Study the drawing (mm; zero at the part's minimum x, y, z) and answer. A direction names the side the tool comes from. Round coordinates to 2 decimals unless told otherwise and drop trailing zeros. Order: outer loops, then holes, each group sorted by start corner. A loop starts at its lowest first (then second) coordinate and runs counter-clockwise, first axis right, second up. Notation, with made-up numbers: (13.25, 81.5) - (33.25, 81.5) arc R32 ccw to (33.25, 118.5) - close; hole circle Ø4 at (87, 50.5). An arc over 180 degrees is marked (long way). Put each result on its own line as item: value.
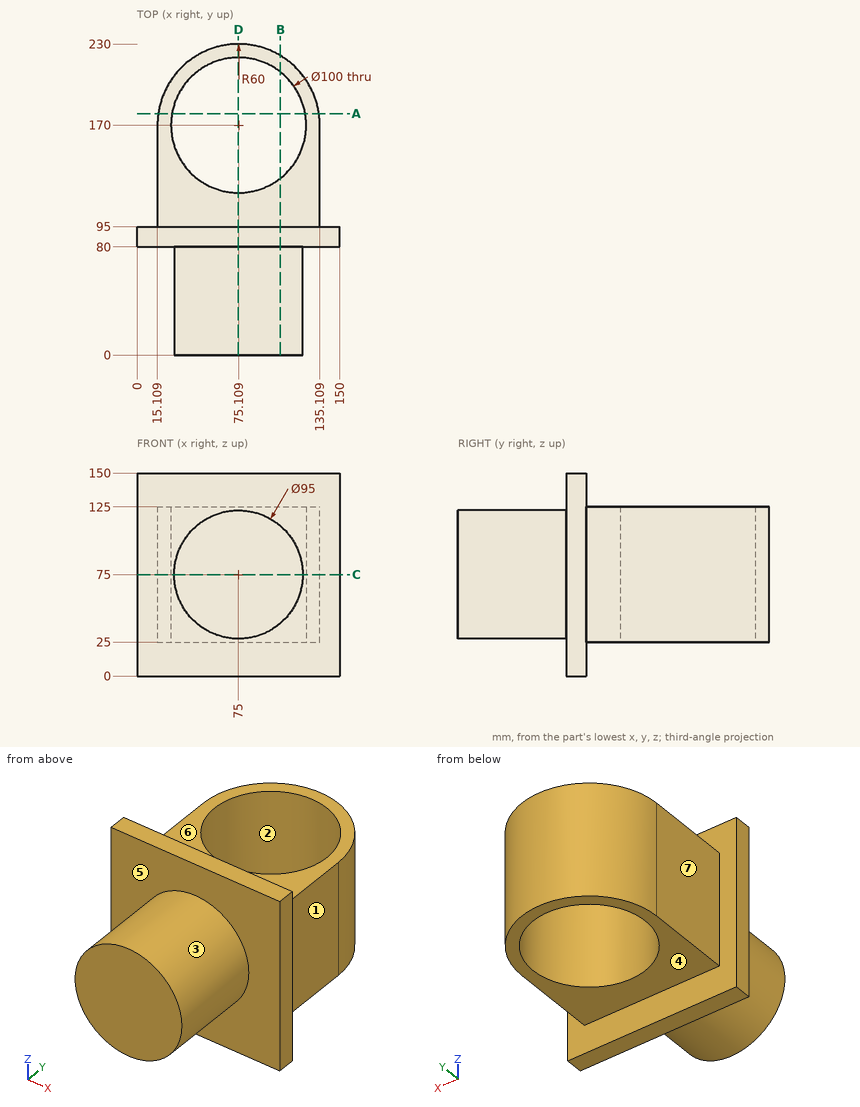
1) A cutting plane is placed at C-C on z = 75. Write down the section's boundary in (x, y), then the cut area to 3 significant figures.
Findings below:
outline: (0, 80) - (27.5, 80) - (27.5, 0) - (122.5, 0) - (122.5, 80) - (150, 80) - (150, 95) - (135.11, 95) - (135.11, 170) arc R60 ccw to (15.11, 170) - (15.11, 95) - (0, 95) - close; hole circle Ø100 at (75.11, 170)
area: 16,700 mm2
2) A cutting plane is placed at A-A on y = 178.5. Write down the section's boundary in (x, z).
Findings below:
outline: (15.71, 25) - (25.84, 25) - (25.84, 125) - (15.71, 125) - close; (124.38, 25) - (134.5, 25) - (134.5, 125) - (124.38, 125) - close
3) A cutting plane is placed at B-B on x = 106. Write down the section's boundary in (y, z).
Findings below:
outline: (0, 39.01) - (80, 39.01) - (80, 0) - (95, 0) - (95, 25) - (130.68, 25) - (130.68, 125) - (95, 125) - (95, 150) - (80, 150) - (80, 110.99) - (0, 110.99) - close; (209.32, 25) - (221.44, 25) - (221.44, 125) - (209.32, 125) - close
4) For the marked faces 5, 6 and 7, determine the directions among +Z, -Z, +X, -X, +Y, -Y from which every point of the face is accessible in a straight line to the end or side of a thin tool.
Findings below:
face 5: -Y
face 6: +Z, +X, -X, +Y
face 7: +Z, -Z, -X, +Y
5) For a pull along X with two mould halves and no side action, classify the marked faces 1, 2, 3 and 4 as pulls with the +X half, pulls with the -X half, needs draft (parallel to the pull), parting line crosses it, or undercut.
Findings below:
face 1: pulls with the +X half
face 2: undercut
face 3: parting line crosses it
face 4: needs draft
6) A cutting plane is placed at D-D on x = 75. Write down the section's boundary in (y, z), then the cut area to 4 significant figures.
Findings below:
outline: (0, 27.5) - (80, 27.5) - (80, 0) - (95, 0) - (95, 25) - (120, 25) - (120, 125) - (95, 125) - (95, 150) - (80, 150) - (80, 122.5) - (0, 122.5) - close; (220, 25) - (230, 25) - (230, 125) - (220, 125) - close
area: 13,350 mm2
7) Straight lines are drawn through the part: L1, parallel to Y at x = 98.5, z = 136.5; L2, parallel to Z at x = 24.5, y = 157.5; L3, parallel to Y at x = 87.5, z = 87. For each, find the intervals that lie inside material, in ascending order. Write a range as from..to.
Findings below:
L1: y = 80..95
L2: z = 25..125
L3: y = 0..121.56, 218.44..228.71
8) Given pin 1 Ø1.5 at (x, z) = (111.5, 15.5) entering from +Y; pin 2 Ø10 at (x, y) = (42.5, 133.5) entering from +Z; pin 3 Ø1 at (y, z) = (170, 83) entering from -X, each flat-ended and moving along its own axis, determine where each tip first touches the part or whether it passes through.
Findings below:
pin 1: stops at y = 95
pin 2: stops at z = 125
pin 3: stops at x = 15.11
